```python
from build123d import *

# Parameters (mm, degrees)
SCALE1_SCALE        = 6
SKETCH4_R           = 45.852
BOSS_EXTRUDE1_DEPTH = 12.7
SKETCH5_R           = 27
CUT_EXTRUDE1_DEPTH  = 84.317043923
SCALE2_SCALE        = 3.323882225
SKETCH7_R           = 152.406647765
SKETCH7_R_2         = 89.744820066
BOSS_EXTRUDE2_DEPTH = 33.99
SCALE3_SCALE        = 0.416652997
BOSS_EXTRUDE3_START = -31.75
SKETCH8_R           = 76.200686546
BOSS_EXTRUDE3_DEPTH = 12.7
SKETCH9_R           = 63.500686546
SKETCH9_R_2         = 37.392448241
BOSS_EXTRUDE4_DEPTH = 19.05
SKETCH10_R          = 37.392448241
CUT_EXTRUDE2_DEPTH  = 137.337641642
SCALE4_SCALE        = 0.70539227
SKETCH11_R          = 44.792893449
SKETCH11_R_2        = 26.376343957
BOSS_EXTRUDE5_DEPTH = 41.32
SCALE5_SCALE        = 0.666666667


with BuildPart() as part:
    # Sketch1 → Revolve1 (revolve)
    with BuildSketch(Plane.XY, mode=Mode.PRIVATE) as revolve1_sk:
        with BuildLine():
            Line((0, 0), (4, 0))
            Line((4, 0), (4, 3.142))
            Line((4, 3.142), (1.9, 3.142))
            ThreePointArc((1.9, 3.142), (0, 2.051053651), (-1.9, 3.142))
            Line((-1.9, 3.142), (-4, 3.142))
            Line((-4, 3.142), (-4, 0))
            Line((-4, 0), (0, 0))
        make_face()
    revolve(revolve1_sk.sketch.rotate(Axis((-4, -4.5, 0), (1, 0, 0)), 90), axis=Axis((-4, -4.5, 0), (1, 0, 0)))


with BuildPart() as part_1:
    # Scale1: scaled about (0, -4.5, 0)
    add(part.part.scale(SCALE1_SCALE).moved(Location((0, 22.5, 0))))

    # Sketch4 → Boss-Extrude1 (add)
    with BuildSketch(Plane(origin=(24, 0, 0), x_dir=(0, 0, -1), z_dir=(1, 0, 0))):
        with Locations(Location((0, -4.5, 0), (0, 0, 180))):
            Circle(SKETCH4_R)
    extrude(amount=BOSS_EXTRUDE1_DEPTH)

    # Sketch5 → Cut-Extrude1 (cut, through all)
    with BuildSketch(Plane.ZY.offset(-24)):
        with Locations((0, -4.5)):
            Circle(SKETCH5_R)
    extrude(amount=-CUT_EXTRUDE1_DEPTH, mode=Mode.SUBTRACT)


with BuildPart() as part_2:
    # Scale2: scaled about (7.131190873, -4.5, 0)
    add(part_1.part.scale(SCALE2_SCALE).moved(Location((-16.57204771, 10.457470011, 0))))

    # Sketch7 → Boss-Extrude2 (add)
    with BuildSketch(Plane(origin=(105.414429934, 0, 0), x_dir=(0, 0, -1), z_dir=(1, 0, 0))):
        with Locations(Location((0, -4.5, 0), (0, 0, 180))):
            Circle(SKETCH7_R)
        with Locations(Location((0, -4.5, 0), (0, 0, 180))):
            Circle(SKETCH7_R_2, mode=Mode.SUBTRACT)
    extrude(amount=BOSS_EXTRUDE2_DEPTH)


with BuildPart() as part_3:
    # Scale3: scaled about (25.471225568, -4.5, 0)
    add(part_2.part.scale(SCALE3_SCALE).moved(Location((14.858563099, -2.625061514, 0))))

    # Sketch8 → Boss-Extrude3 (add)
    with BuildSketch(Plane(origin=(72.941836619, 0, 0), x_dir=(0, 0, -1), z_dir=(1, 0, 0)).offset(BOSS_EXTRUDE3_START)):
        with Locations((0, -4.5)):
            Circle(SKETCH8_R)
    extrude(amount=BOSS_EXTRUDE3_DEPTH)

    # Sketch9 → Boss-Extrude4 (add)
    with BuildSketch(Plane(origin=(72.941836619, 0, 0), x_dir=(0, 0, -1), z_dir=(1, 0, 0))):
        with Locations(Location((0, -4.5, 0), (0, 0, 180))):
            Circle(SKETCH9_R)
        with Locations(Location((0, -4.5, 0), (0, 0, 180))):
            Circle(SKETCH9_R_2, mode=Mode.SUBTRACT)
    extrude(amount=BOSS_EXTRUDE4_DEPTH)

    # Sketch10 → Cut-Extrude2 (cut, through all)
    with BuildSketch(Plane(origin=(53.891836619, 0, 0), x_dir=(0, 0, -1), z_dir=(1, 0, 0))):
        with Locations(Location((0, -4.5, 0), (0, 0, 180))):
            Circle(SKETCH10_R)
    extrude(amount=-CUT_EXTRUDE2_DEPTH, mode=Mode.SUBTRACT)


with BuildPart() as part_4:
    # Scale4: scaled about (36.400291081, -4.5, 0)
    add(part_3.part.scale(SCALE4_SCALE).moved(Location((10.723807116, -1.325734784, 0))))

    # Sketch11 → Boss-Extrude5 (add)
    with BuildSketch(Plane(origin=(75.614137598, 0, 0), x_dir=(0, 0, -1), z_dir=(1, 0, 0))):
        with Locations(Location((0, -4.5, 0), (0, 0, 180))):
            Circle(SKETCH11_R)
        with Locations(Location((0, -4.5, 0), (0, 0, 180))):
            Circle(SKETCH11_R_2, mode=Mode.SUBTRACT)
    extrude(amount=BOSS_EXTRUDE5_DEPTH)


with BuildPart() as part_5:
    # Scale5: scaled about (56.419036868, -4.5, 0)
    add(part_4.part.scale(SCALE5_SCALE).moved(Location((18.806345623, -1.5, 0))))


solid = part_5.part
```
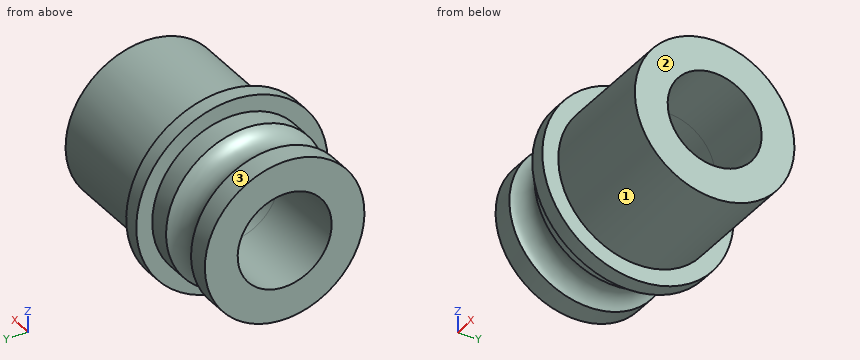
Source: CAD feature listing. Evaluate the final solid. Frame: model axes, mm. Face numbers are marked on the shaded views. A direction names the side the tool comes from. Round coordinates to 2 decimals unless told otherwise and drop trailing zeros. Loops run counter-clockwise (first coordinate to the right, second up) from the corner with the lowest first, then second, coordinate; pieces in that order, holes last.
(1) Contact query for flat-ended pins moving along their axis: pin 1 Ø6 at (x, z) = (32.5, 18) entering from -Y; pin 2 Ø10 at (x, z) = (47.5, 25) entering from +Y; pin 3 Ø5 at (x, y) = (57.5, -30.5) entering from +Z; pin 4 Ø1.5 at (y, z) = (-30, 16) entering from +X. Output: stop coordinate, or through.
From the geometry:
pin 1: stops at y = -26.54
pin 2: stops at y = 25.23
pin 3: stops at z = 18.43
pin 4: stops at x = 96.76
(2) Access query for the marked faces 1, 2 and 3. Directions: +Z, -Z, +X, -X, +Y, -Y. A direction counts if a zero-diameter tool reaches every point of the face in a straight line with its end or side. Return the directions, or none.
From the geometry:
face 1: +X
face 2: +Z, -Z, +X, +Y, -Y
face 3: -X
(3) Section query B-B (x = 80). Output: boundary loops of the cut face in (y, z), and give its area (3 significant figures).
From the geometry:
outline: circle Ø59.72 at (-4.5, 0); hole circle Ø35.17 at (-4.5, 0)
area: 1,830 mm2
(4) Section query A-A (z = 0). Output: boundary loops of the cut face in (x, y), and give its area (3 significant figures).
From the geometry:
outline: (14.07, -34.36) - (22.27, -34.36) arc R8.6 cw to (37.12, -34.36) - (45.33, -34.36) - (45.33, -40.33) - (51.3, -40.33) - (51.3, -34.36) - (96.76, -34.36) - (96.76, -22.08) - (14.07, -22.08) - close; (14.07, 13.08) - (96.76, 13.08) - (96.76, 25.36) - (51.3, 25.36) - (51.3, 31.33) - (45.33, 31.33) - (45.33, 25.36) - (37.12, 25.36) arc R8.6 cw to (22.27, 25.36) - (14.07, 25.36) - close
area: 2,010 mm2
(5) Material intervals for probe 1 along Z at (x, y) = (48.15, -4.5); probe 2 along Z at (x, y) = (56, -4); probe 3 along X at (y, z) = (-3.5, 29.5), sorted ascending.
From the geometry:
probe 1: z = -35.83 to -17.58, 17.58 to 35.83
probe 2: z = -29.86 to -17.58, 17.58 to 29.86
probe 3: x = 14.07 to 22.48, 36.91 to 96.76
